Input: part model. Units: mm. Frame: model coordinates. A direction names the side the tool comes from. Round coordinates to 2 decimals unless told otherwise and drop trailing zeros. Loops run counter-clockwise (first coordinate to the right, second up) from the corner with the lowest first, then second, coordinate; pieces in that order, holes last. Notation, with made-up numbers: (-13, -37) -> (-5, -37) arc R19 cw to (-5, -29) -> close; hole circle Ø7 at (49.5, 69.5). An arc over 180 degrees is marked (long way). Answer as a JSON object with one key per item and string values. Group by question number.
Item 1: Section query C-C on x = -52. Return loops of the section in (y, z).
Item 2: Section query D-D on z = 29.5. Return loops of the section in (x, y), and give its area (3 significant figures).
Item 3: Pin query (flat end, axial travel): pin 1 (2.5 mm diameter, centred on x = 15.5, z = 15.5, fed in from -Y); pin 2 (4 mm diameter, centred on x = -42, y = 28.5, fed in from -Z); pin 3 (3 mm diameter, centred on y = 58, z = -48, fed in from +X). Return the tip coordinate at first contact, or that it passes through.
Item 4: Section query A-A on x = 0. Return loops of the section in (y, z).
Item 5: Set-up query: faces 4 (the flat face through (-13, 8, 13)), 5 (the cylindrical face through (2.75, 3.94, -62.44)), 6 (the cylindrical face through (15.43, 3.94, 14)). Return all of +Z, -Z, +X, -X, +Y, -Y with unobstructed straight access to the full face (end or side cutting, diameter ignored); none if empty.
Item 6: Material intervals for line 1 (Y direction, x = -17, z = -1.5); line 2 (X direction, y = 4.5, z = 15.5); line 3 (X direction, y = 3, z = 0), sorted ascending. Write a range as [from, to].
Item 7: Section query B-B on z = -5. Return loops of the section in (x, y), and give its area (3 significant figures).
Item 8: Draft query along Y for faces 1 (the flat face through (-13, 0, 13)), 2 (the cylindrical face through (-15.43, 3.94, 17)), 3 (the cylindrical face through (-38.671, 32.65, -43.886)). Return one class per face: released by +Y, released by -Y, zero draft, split by the parting line, or undercut.
from build123d import *

# Parameters (mm, degrees)
SKETCH_2_R          = 62.5
EXTRUDE_1_DEPTH     = 8
SKETCH_3_R          = 5
EXTRUDE_2_DEPTH     = 50
SKETCH_4_R          = 62.5
EXTRUDE_3_DEPTH     = 8
CUT_EXTRUDE_1_REACH = 112.311
SKETCH_5_R          = 15
CUT_EXTRUDE_2_REACH = 112.311
SKETCH_6_R          = 1.5


with BuildPart() as part:
    # 草图2 → 凸台-拉伸1 (new body)
    with BuildSketch(Plane(origin=(0, 0, 0), x_dir=(1, 0, 0), z_dir=(0, 1, 0))):
        with Locations(Location((0, 0, 0), (0, 0, 270))):
            Circle(SKETCH_2_R)
    extrude(amount=EXTRUDE_1_DEPTH)

    # 草图3 → 凸台-拉伸2 (add)
    with BuildSketch(Plane(origin=(0, 8, 0), x_dir=(1, 0, 0), z_dir=(0, 1, 0))):
        with Locations(Location((38.890872965, 38.890872965, 0), (0, 0, 270))):
            Circle(SKETCH_3_R)
        with Locations(Location((38.890872965, -38.890872965, 0), (0, 0, 270))):
            Circle(SKETCH_3_R)
        with Locations(Location((-38.890872965, -38.890872965, 0), (0, 0, 270))):
            Circle(SKETCH_3_R)
        with Locations(Location((-38.890872965, 38.890872965, 0), (0, 0, 270))):
            Circle(SKETCH_3_R)
    extrude(amount=EXTRUDE_2_DEPTH)

    # 草图4 → 凸台-拉伸3 (add)
    with BuildSketch(Plane(origin=(0, 58, 0), x_dir=(1, 0, 0), z_dir=(0, 1, 0))):
        with Locations(Location((0, 0, 0), (0, 0, 270))):
            Circle(SKETCH_4_R)
    extrude(amount=EXTRUDE_3_DEPTH)

    # 草图5 → 切除-拉伸1 (cut, up to next)
    with BuildSketch(Plane.XZ, mode=Mode.PRIVATE) as cut_extrude_1_sk1:
        with Locations(Location((0, 0, 0), (0, 0, 270))):
            Circle(SKETCH_5_R)
    cut_extrude_1_tool1 = extrude(cut_extrude_1_sk1.sketch, amount=-CUT_EXTRUDE_1_REACH, mode=Mode.PRIVATE) & part.part
    add(cut_extrude_1_tool1.solids().sort_by_distance((0, 0, 0))[0], mode=Mode.SUBTRACT)

    # 草图6 → 切除-拉伸2 (cut, up to next)
    with BuildSketch(Plane(origin=(0, 0, 0), x_dir=(-1, 0, 0), z_dir=(0, -1, 0)), mode=Mode.PRIVATE) as cut_extrude_2_sk1:
        with Locations(Location((15.5, -15.5, 0), (0, 0, 90))):
            Circle(SKETCH_6_R)
    cut_extrude_2_tool1 = extrude(cut_extrude_2_sk1.sketch, amount=-CUT_EXTRUDE_2_REACH, mode=Mode.PRIVATE) & part.part
    # 草图6 → 切除-拉伸2 (cut, up to next)
    with BuildSketch(Plane(origin=(0, 0, 0), x_dir=(-1, 0, 0), z_dir=(0, -1, 0)), mode=Mode.PRIVATE) as cut_extrude_2_sk2:
        with Locations(Location((15.5, 15.5, 0), (0, 0, 270))):
            Circle(SKETCH_6_R)
    cut_extrude_2_tool2 = extrude(cut_extrude_2_sk2.sketch, amount=-CUT_EXTRUDE_2_REACH, mode=Mode.PRIVATE) & part.part
    # 草图6 → 切除-拉伸2 (cut, up to next)
    with BuildSketch(Plane(origin=(0, 0, 0), x_dir=(-1, 0, 0), z_dir=(0, -1, 0)), mode=Mode.PRIVATE) as cut_extrude_2_sk3:
        with Locations(Location((-15.5, -15.5, 0), (0, 0, 270))):
            Circle(SKETCH_6_R)
    cut_extrude_2_tool3 = extrude(cut_extrude_2_sk3.sketch, amount=-CUT_EXTRUDE_2_REACH, mode=Mode.PRIVATE) & part.part
    # 草图6 → 切除-拉伸2 (cut, up to next)
    with BuildSketch(Plane(origin=(0, 0, 0), x_dir=(-1, 0, 0), z_dir=(0, -1, 0)), mode=Mode.PRIVATE) as cut_extrude_2_sk4:
        with Locations(Location((-15.5, 15.5, 0), (0, 0, 90))):
            Circle(SKETCH_6_R)
    cut_extrude_2_tool4 = extrude(cut_extrude_2_sk4.sketch, amount=-CUT_EXTRUDE_2_REACH, mode=Mode.PRIVATE) & part.part
    add(cut_extrude_2_tool1.solids().sort_by_distance((-15.5, 0, 15.5))[0], mode=Mode.SUBTRACT)
    add(cut_extrude_2_tool2.solids().sort_by_distance((-15.5, 0, -15.5))[0], mode=Mode.SUBTRACT)
    add(cut_extrude_2_tool3.solids().sort_by_distance((15.5, 0, 15.5))[0], mode=Mode.SUBTRACT)
    add(cut_extrude_2_tool4.solids().sort_by_distance((15.5, 0, -15.5))[0], mode=Mode.SUBTRACT)


solid = part.part
Solved:
{
 "1": {"outline": "(0, -34.67) -> (8, -34.67) -> (8, 34.67) -> (0, 34.67) -> close; (58, -34.67) -> (66, -34.67) -> (66, 34.67) -> (58, 34.67) -> close"},
 "2": {"outline": "(-55.1, 0) -> (55.1, 0) -> (55.1, 8) -> (-55.1, 8) -> close; (-55.1, 58) -> (55.1, 58) -> (55.1, 66) -> (-55.1, 66) -> close", "area": "1,760 mm²"},
 "3": {"pin 1": "y = 58", "pin 2": "z = -43.77", "pin 3": "x = 41.76"},
 "4": {"outline": "(0, -62.5) -> (8, -62.5) -> (8, -15) -> (0, -15) -> close; (0, 15) -> (8, 15) -> (8, 62.5) -> (0, 62.5) -> close; (58, -62.5) -> (66, -62.5) -> (66, 62.5) -> (58, 62.5) -> close"},
 "5": {"face 4": "none", "face 5": "+Y, -Y", "face 6": "-Y"},
 "6": {"line 1": "[0, 8], [58, 66]", "line 2": "[-60.55, -17], [-14, 14], [17, 60.55]", "line 3": "[-62.5, -15], [15, 62.5]"},
 "7": {"outline": "(-62.3, 0) -> (-14.14, 0) -> (-14.14, 8) -> (-62.3, 8) -> close; (-62.3, 58) -> (62.3, 58) -> (62.3, 66) -> (-62.3, 66) -> close; (14.14, 0) -> (62.3, 0) -> (62.3, 8) -> (14.14, 8) -> close", "area": "1,770 mm²"},
 "8": {"face 1": "released by -Y", "face 2": "zero draft", "face 3": "undercut"}
}
